Verification items for the finished model (mm, model axes). Round coordinates to 2 decimals unless told otherwise and drop trailing zeros. Order: outer loops, then holes, each group sorted by start corner. A loop starts at its lowest first (then second) coordinate and runs counter-clockwise, first axis right, second up.
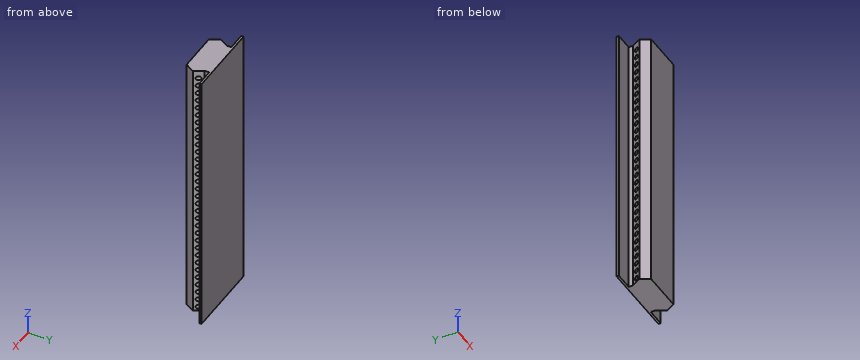
```python
from build123d import *

# Parameters (mm, degrees)
BOSS_EXTRUDE1_DEPTH = 120.69
SKETCH2_R           = 1
CUT_EXTRUDE1_DEPTH  = 123.482966683
LPATTERN1_COUNT     = 32
LPATTERN1_PITCH     = 3.71


with BuildPart() as part:
    # Sketch1 → Boss-Extrude1 (new body)
    with BuildSketch(Plane.XY):
        Polygon((9.693000417, 0), (-8.306999583, 0), (-10.641999583, 4.044338636), (-8.306999583, 8.088677271), (-8.306999583, 10.088677271), (-16.306999583, 10.088677271), (-16.306999583, 11.088677271), (17.693000417, 11.088677271), (17.693000417, 10.088677271), (9.693000417, 10.088677271), (9.693000417, 8.088677271), (12.028000417, 4.044338636), align=None)
    extrude(amount=-BOSS_EXTRUDE1_DEPTH)

    # Sketch2 → Cut-Extrude1 (cut, symmetric)
    with BuildSketch(Plane(origin=(0, 0, 0), x_dir=(0, 0, -1), z_dir=(1, 0, 0))):
        with Locations(Location((3.71, 5.988677271, 0), (0, 0, 90))):
            Circle(SKETCH2_R)
    cut_extrude1 = extrude(amount=CUT_EXTRUDE1_DEPTH, both=True, mode=Mode.SUBTRACT)

    # LPattern1: Cut-Extrude1 ×32
    with Locations(*[(0, 0, -i * LPATTERN1_PITCH) for i in range(1, LPATTERN1_COUNT)]):
        add(cut_extrude1, mode=Mode.SUBTRACT)


solid = part.part
```
1) Scan lines: probe 1 along Y at (x, z) = (2.75, -51.94); probe 2 along Y at (x, z) = (-12, -59.5); probe 3 along Y at (x, z) = (-1, -111). Record each from-to range of solid material in increasing order.
2) Sectioned sample at B-B on x = 4. Count the separate pieces of the cut face and the enclosed holes in it, then the cut area to 3 significant figures.
3) Sectioned sample at A-A on x = -13. Record the cut outline in (y, z).
4) Go/stop test with flat-tipped pins: pin 1 Ø1.8 at (y, z) = (5.99, -85.33) entering from -X; pin 2 Ø2 at (y, z) = (8.5, -89) entering from +X; pin 3 Ø2.5 at (y, z) = (5.99, -48.23) entering from +X; pin 4 Ø12 at (x, z) = (10, -20.5) entering from -Y. Record where each tip stops, or that it passes through.
5) Sectioned sample at C-C on y = 2.25. Record the cut outline in (x, z), then the cut area to 3 significant figures.
Returned:
1. probe 1: y = 0 to 4.99, 6.99 to 11.09
1. probe 2: y = 10.09 to 11.09
1. probe 3: y = 0 to 5.03, 6.94 to 11.09
2. separate pieces: 1
2. enclosed holes: 32
2. area: 1,240 mm2
3. outline: (10.09, -120.69) - (11.09, -120.69) - (11.09, 0) - (10.09, 0) - close
4. pin 1: passes through
4. pin 2: stops at x = 10.03
4. pin 3: stops at x = 11.63
4. pin 4: stops at y = 0
5. outline: (-9.61, -120.69) - (10.99, -120.69) - (10.99, 0) - (-9.61, 0) - close
5. area: 2,490 mm2
